```python
from build123d import *

# Parameters (mm, degrees)
AUFSATZ_LINEAR_AUSTRAGEN1_DEPTH = 10
SKIZZE2_R                       = 1.75
SCHNITT_LINEAR_AUSTRAGEN1_DEPTH = 36.05
SKIZZE4_R                       = 2.25
SCHNITT_LINEAR_AUSTRAGEN3_DEPTH = 50.25
VERRUNDUNG1_R                   = 10
SCHNITT_LINEAR_AUSTRAGEN5_DEPTH = 11
FASE1_SIZE                      = 1.5
SCHNITT_LINEAR_AUSTRAGEN6_DEPTH = 11


with BuildPart() as part:
    # Skizze1 → Aufsatz-Linear austragen1 (new body)
    with BuildSketch(Plane.XY):
        with BuildLine():
            Line((0.5, -26.545291485), (0.5, -30.545908073))
            Line((0.5, -30.545908073), (0.5, -37.545908073))
            Line((0.5, -37.545908073), (4.5, -37.545908073))
            Line((4.5, -37.545908073), (4.5, -30.216758595))
            ThreePointArc((4.5, -30.216758595), (29.558680329, -7.719256261), (18.7, 24.158073185))
            Line((18.7, 24.158073185), (18.7, 51.55))
            Line((18.7, 51.55), (10.2, 51.55))
            Line((10.2, 51.55), (10.2, 31.55))
            Line((10.2, 31.55), (-10.2, 31.55))
            Line((-10.2, 31.55), (-10.2, 51.55))
            Line((-10.2, 51.55), (-18.7, 51.55))
            Line((-18.7, 51.55), (-18.7, 24.158073185))
            ThreePointArc((-18.7, 24.158073185), (-29.558680329, -7.719256261), (-4.5, -30.216758595))
            Line((-4.5, -30.216758595), (-4.5, -37.545908073))
            Line((-4.5, -37.545908073), (-0.5, -37.545908073))
            Line((-0.5, -37.545908073), (-0.5, -30.545908073))
            Line((-0.5, -30.545908073), (-0.5, -26.545291485))
            ThreePointArc((-0.5, -26.545291485), (0, 26.55), (0.5, -26.545291485))
        make_face()
    extrude(amount=AUFSATZ_LINEAR_AUSTRAGEN1_DEPTH)

    # Skizze2 → Schnitt-Linear austragen1 (cut, through all)
    with BuildSketch(Plane.ZY.offset(4.5)):
        with Locations((5, -33.881333334)):
            Circle(SKIZZE2_R)
    extrude(amount=-SCHNITT_LINEAR_AUSTRAGEN1_DEPTH, mode=Mode.SUBTRACT)

    # Skizze4 → Schnitt-Linear austragen3 (cut, through all)
    with BuildSketch(Plane.ZY.offset(18.7)):
        with Locations((5, 41.55)):
            Circle(SKIZZE4_R)
    extrude(amount=-SCHNITT_LINEAR_AUSTRAGEN3_DEPTH, mode=Mode.SUBTRACT)

    # Verrundung1
    verrundung1_edges = [part.edges().sort_by_distance(p)[0] for p in [
        (-18.7, 24.158073185, 5),
        (18.7, 24.158073185, 5),
    ]]
    fillet(verrundung1_edges, radius=VERRUNDUNG1_R)

    # Skizze6 → Schnitt-Linear austragen5 (cut, through all)
    with BuildSketch(Plane.XY):
        Polygon((0, 0), (0, 63.91348789), (40.013946788, 63.91348789), (48.360414216, -54.819102682), (0, -54.819102682), align=None)
    extrude(amount=SCHNITT_LINEAR_AUSTRAGEN5_DEPTH, mode=Mode.SUBTRACT)

    # Fase1
    fase1_edges = [part.edges().sort_by_distance(p)[0] for p in [
        (-18.7, 40.098167422, 0),
        (-18.7, 40.098167422, 10),
        (-29.006358008, -9.588206043, 0),
        (-29.006358008, -9.588206043, 10),
        (-19.459415096, 24.823823807, 0),
        (-19.459415096, 24.823823807, 10),
    ]]
    chamfer(fase1_edges, length=FASE1_SIZE)

    # Skizze7 → Schnitt-Linear austragen6 (cut, through all)
    with BuildSketch(Plane.XY.offset(10)):
        Polygon((1.325, 29.05), (0, 29.05), (0, 31.55), (-0.15, 31.55), (-0.15, 29.05), (-1.325, 29.05), (-1.325, 25.137104209), (1.325, 25.137104209), align=None)
    extrude(amount=-SCHNITT_LINEAR_AUSTRAGEN6_DEPTH, mode=Mode.SUBTRACT)


solid = part.part
```
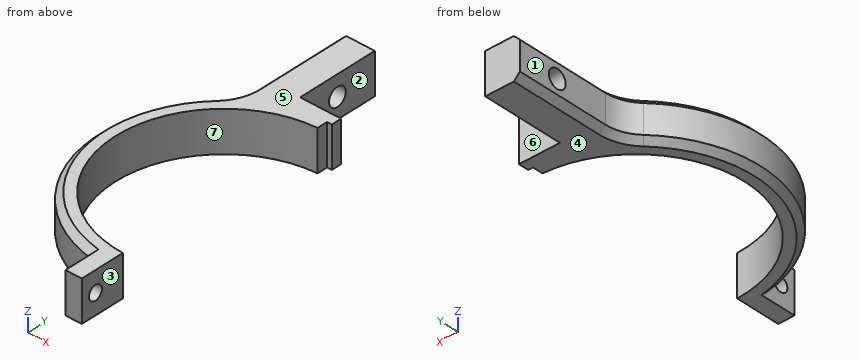
Model file for the job. Use its own axes, mm. Face numbers are marked on the shaded views. A direction names the side the tool comes from. Round coordinates to 2 decimals unless told otherwise and drop trailing zeros. Write each loop counter-clockwise with the first axis right and the second up, starting at its lowest first coordinate (ties: lowest second). Pieces come first, ordered by that corner, then holes. Notation, with made-up numbers: (15, 76) -> (20, 76) arc R9 cw to (20, 88) -> close; hole circle Ø10 at (14, 78.5). An arc over 180 degrees is marked (long way). Answer as CSV lines item,"result".
1. Slice it at B-B, the plane z = 5. List the corners of the cut face in (x, y) (3 decimals), plus the area to 3 significant figures.
Resolved:
outline,"(-21.622, 21.582) arc R30.55 ccw to (-4.5, -30.217) -> (-4.5, -32.131) -> (-0.5, -32.131) -> (-0.5, -26.545) arc R26.55 cw to (-1.325, 26.517) -> (-1.325, 29.05) -> (-0.15, 29.05) -> (-0.15, 31.55) -> (-10.2, 31.55) -> (-10.2, 39.3) -> (-18.7, 39.3) -> (-18.7, 28.646) arc R10 cw to start; (-18.7, 43.8) -> (-10.2, 43.8) -> (-10.2, 51.55) -> (-18.7, 51.55) -> close; (-4.5, -37.546) -> (-0.5, -37.546) -> (-0.5, -35.631) -> (-4.5, -35.631) -> close"
area,"559 mm²"
2. Mould opens along Y. For the marked faces 5, 6 and 7 say: +Y half, -Y half, draft (parallel to the pull), parting line (faces both ways), or undercut.
Resolved:
face 5,"draft"
face 6,"+Y half"
face 7,"undercut"
3. Pin check, flat tips, straight feed: pin 1 Ø4 at (y, z) = (-33.88, 5) entering from +X; pin 2 Ø5 at (y, z) = (45, 6) entering from +X; pin 3 Ø1 at (y, z) = (-20.5, 1) entering from -X. Stop position of each tip, or through.
Resolved:
pin 1,"x = -0.5"
pin 2,"x = -10.2"
pin 3,"x = -22.79"
4. Drill centre lines: line 1 (Y direction, x = -15.5, z = 5); line 2 (Y direction, x = -2.5, z = 4.5); line 3 (X direction, y = 33.5, z = 1.5). Where is each one in solid material? Low to high.
Resolved:
line 1,"-26.33 to -21.56, 21.56 to 39.3, 43.8 to 51.55"
line 2,"-37.55 to -35.56, -32.2 to -26.43, 26.43 to 31.55"
line 3,"-18.7 to -10.2"
5. Slice it at A-A, the plane y = 41.55. List the corners of the cut face in (x, z), plus the area to 3 significant figures.
Resolved:
outline,"(-18.7, 1.5) -> (-17.2, 0) -> (-10.2, 0) -> (-10.2, 2.75) -> (-18.7, 2.75) -> close; (-18.7, 7.25) -> (-10.2, 7.25) -> (-10.2, 10) -> (-17.2, 10) -> (-18.7, 8.5) -> close"
area,"44.5 mm²"
6. Tool access for the marked faces 1, 2, 3 and 4: list every direction of +Z, -Z, +X, -X, +Y, -Y with a clear straight run to the whole face (end or side of a thin tool).
Resolved:
face 1,"+Z, -Z, -X, +Y"
face 2,"+Z, -Z, +X, +Y"
face 3,"+Z, -Z, +X, -Y"
face 4,"-Z, +X, -X, +Y, -Y"
7. Slice it at D-D, the plane y = -31. List the corners of the cut face in (x, z), plus the area to 3 significant figures.
Resolved:
outline,"(-4.5, 0) -> (-0.5, 0) -> (-0.5, 10) -> (-4.5, 10) -> close"
area,"40.0 mm²"
8. Slice it at C-C, the plane y = 0. List the corners of the cut face in (x, z).
Resolved:
outline,"(-30.55, 1.5) -> (-29.05, 0) -> (-26.55, 0) -> (-26.55, 10) -> (-29.05, 10) -> (-30.55, 8.5) -> close"
